from build123d import *

# Parameters (mm, degrees)
SKETCH1_W           = 40
SKETCH1_H           = 30
BOSS_EXTRUDE1_DEPTH = 2
BOSS_EXTRUDE2_DEPTH = 4


with BuildPart() as part:
    # Sketch1 → Boss-Extrude1 (new body)
    with BuildSketch(Plane.XY):
        Rectangle(SKETCH1_W, SKETCH1_H)
    extrude(amount=BOSS_EXTRUDE1_DEPTH)

    # Sketch2 → Boss-Extrude2 (add)
    with BuildSketch(Plane.XY.offset(2)):
        Polygon((-0.128668655, 9.175508535), (1.807002834, 2.884576195), (8.823811983, 2.642617259), (3.500715387, -1.954602529), (5.436386876, -8.245534869), (-0.370627592, -4.37419189), (-5.693724187, -8.245534869), (-3.758052698, -1.954602529), (-9.081149293, 2.642617259), (-2.064340145, 2.884576195), align=None)
    extrude(amount=BOSS_EXTRUDE2_DEPTH)


solid = part.part
Read the model definition and answer for the solid it produces. Units are mm, in the model's axes. A direction names the side the tool comes from. Coordinates: 2 decimals unless noted, no trailing zeros. Loops run counter-clockwise (first coordinate to the right, second up) from the corner with the lowest first, then second, coordinate; pieces in that order, holes last. Notation, with made-up numbers: (24, 37.25) - (65, 37.25) arc R20 cw to (65, 70.25) - close; hole circle Ø4 at (34.25, 34). An arc over 180 degrees is marked (long way). Answer in a Markdown table with one row per item.
Q1. Given P1, Ø10, axis at x = 6, y = 8.5, coming from the +Z side, flat-ended and moving along its own axis, determine where the tip first touches the part or whether it passes through.
Here are the results:
| item | result |
|---|---|
| P1 | stops at z = 2 |
Q2. Find section B-B on x = -6.5. Write down the section's boundary in (y, z), plus the area to 3 significant figures.
Here are the results:
| item | result |
|---|---|
| outline | (-15, 0) - (15, 0) - (15, 2) - (2.73, 2) - (2.73, 6) - (0.41, 6) - (0.41, 2) - (-15, 2) - close |
| area | 69.3 mm^2 |
Q3. Straight lines are drawn through the part: line 1 along Z through (x, y) = (14, -13.25); line 2 along X through (y, z) = (-5.25, 4.9); line 3 along Y through (x, z) = (2.5, 5.6). For each, find the intervals that lie inside material, in ascending order. Write a range as [from, to].
Here are the results:
| item | result |
|---|---|
| line 1 | z = [0, 2] |
| line 2 | x = [-4.77, -1.57], [0.94, 4.51] |
| line 3 | y = [-6.29, 2.86] |
Q4. For faces 1 (the flat face through (-2.99, -6.28, 3.97)), 2 (the flat face through (4.455, -5.056, 3.972)), 3 (the flat face through (-1.11, 5.99, 3.97)), determine the directions among +Z, -Z, +X, -X, +Y, -Y from which every point of the face is accessible in a straight line to the end or side of a thin tool.
Here are the results:
| item | result |
|---|---|
| face 1 | +Z, -Y |
| face 2 | +Z, +X |
| face 3 | +Z, -X, +Y |
Q5. Find section C-C on y = 0. Write down the section's boundary in (x, z), plus the area to 3 significant figures.
Here are the results:
| item | result |
|---|---|
| outline | (-20, 0) - (20, 0) - (20, 2) - (5.76, 2) - (5.76, 6) - (-6.02, 6) - (-6.02, 2) - (-20, 2) - close |
| area | 127 mm^2 |
Q6. Find section A-A on z = 4.35. Write down the section's boundary in (x, y), plus the area to 3 significant figures.
Here are the results:
| item | result |
|---|---|
| outline | (-9.08, 2.64) - (-3.76, -1.95) - (-5.69, -8.25) - (-0.37, -4.37) - (5.44, -8.25) - (3.5, -1.95) - (8.82, 2.64) - (1.81, 2.88) - (-0.13, 9.18) - (-2.06, 2.88) - close |
| area | 109 mm^2 |
Q7. The mould has two halves that part along Y. Classify faces 4 (the flat face through (-4.74, -5.14, 3.97)), 5 (the flat face through (2.574, -6.337, 3.972)), 6 (the flat face through (-6.38, 0.31, 3.97)), 7 (the flat face through (20, 0, 1)): pulls with the +Y half, pulls with the -Y half, needs draft (parallel to the pull), parting line crosses it, or undercut.
Here are the results:
| item | result |
|---|---|
| face 4 | undercut |
| face 5 | pulls with the -Y half |
| face 6 | undercut |
| face 7 | needs draft |
